Could you check a few things on this drawing? It's one solid part, dimensions in mm from its lowest x, y, z. Round coordinates to 2 decimals unless told otherwise and drop trailing zeros. Put each result on its own line as item: value.
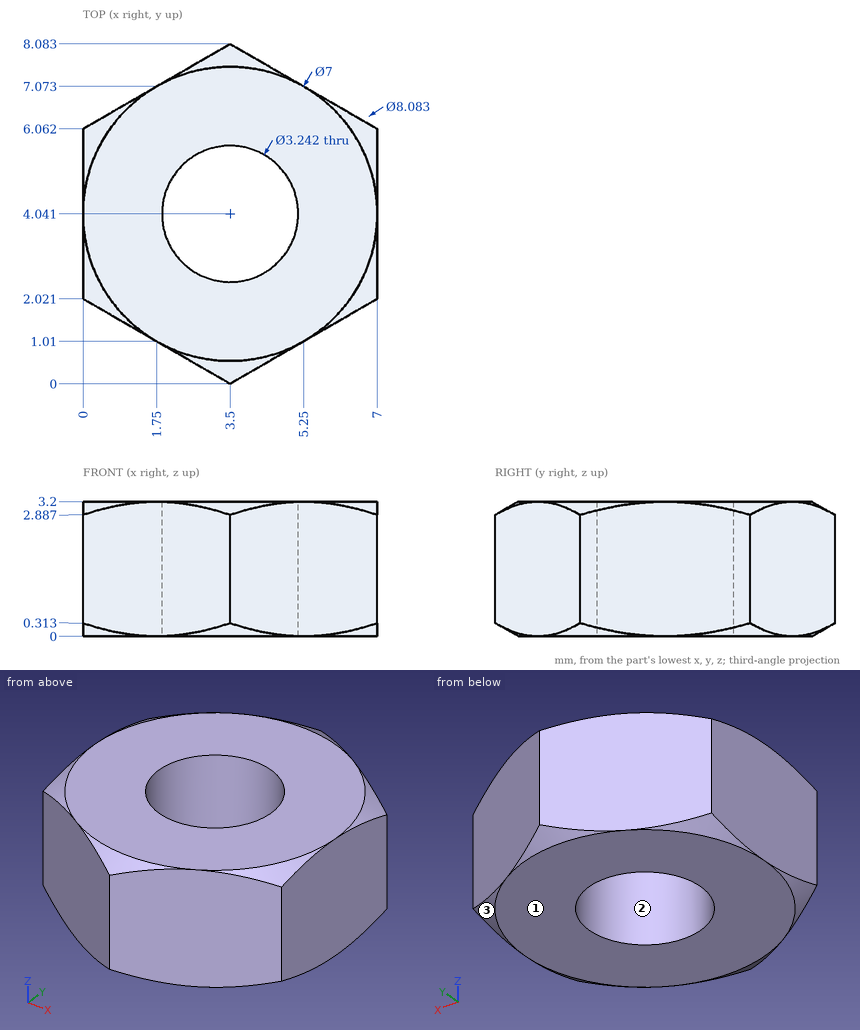
(1) I'm going to push a flat-ended pin straight in: pin 1 (3 mm diameter, centred on x = 2.5, y = 4.5, fed in from -Z). Where does the tip first touch, or does it pass through?
Values found:
pin 1: stops at z = 0
(2) If we mould it in two halves opening along Y, with no side actions, what happens to the marked faces 1, 2 and 3? For each: pulls with the +Y half, pulls with the -Y half, needs draft (parallel to the pull), parting line crosses it, or undercut.
Values found:
face 1: needs draft
face 2: undercut
face 3: pulls with the +Y half
(3) Please list where these lines run through material, in increasing order: probe 1 along Y at (x, z) = (3, 1.55) (1 decimal); probe 2 along X at (y, z) = (4.75, 0.6); probe 3 along X at (y, z) = (5.5, 2.5) (1 decimal). Write a range as from..to.
Values found:
probe 1: y = 0.3..2.5, 5.6..7.8
probe 2: x = 0..2.04, 4.96..7
probe 3: x = 0..2.8, 4.2..7
